from build123d import *

# Parameters (mm, degrees)
SKETCH_1_R      = 1.3
SKETCH_1_R_2    = 4
SKETCH_1_R_3    = 1.925
SKETCH_1_R_4    = 3.85
EXTRUDE_1_DEPTH = 1.5


with BuildPart() as part:
    # 草圖1 → 填料-伸長1 (new body)
    with BuildSketch(Plane(origin=(0, 0, 0), x_dir=(0, 0, -1), z_dir=(1, 0, 0))):
        with BuildLine():
            ThreePointArc((111.555989952, -8.572011863), (6.374730125, -10.137132711), (-98.230068302, -21.244930328))
            ThreePointArc((-98.230068302, -21.244930328), (-123.67575498, -2.873316644), (-103.541794939, 21.20204032))
            ThreePointArc((-103.541794939, 21.20204032), (5.082777822, 20.871677912), (113.584507189, 15.696576829))
            ThreePointArc((113.584507189, 15.696576829), (123.827345593, 3.028727453), (112.406990492, -8.588743688))
            ThreePointArc((112.406990492, -8.588743688), (111.981133536, -8.59851924), (111.555989952, -8.572011863))
        make_face()
        with Locations((-102.143981395, 6.633331517)):
            Circle(SKETCH_1_R, mode=Mode.SUBTRACT)
        with Locations((-108.643981395, 0.133331517)):
            Circle(SKETCH_1_R, mode=Mode.SUBTRACT)
        with Locations((-102.143981395, -6.366668483)):
            Circle(SKETCH_1_R, mode=Mode.SUBTRACT)
        with Locations((-95.643981395, 0.133331517)):
            Circle(SKETCH_1_R, mode=Mode.SUBTRACT)
        with Locations((-102.143981395, 0.133331517)):
            Circle(SKETCH_1_R_2, mode=Mode.SUBTRACT)
        with Locations((35.001055541, 5.982881827)):
            Circle(SKETCH_1_R_3, mode=Mode.SUBTRACT)
        with Locations((-44.432813653, 4.686665047)):
            Circle(SKETCH_1_R_3, mode=Mode.SUBTRACT)
        with Locations((111.605339346, 3.621333032)):
            Circle(SKETCH_1_R_4, mode=Mode.SUBTRACT)
    extrude(amount=EXTRUDE_1_DEPTH)


solid = part.part
Geometry check sheet. Reference: the model listing, model coordinates, mm. A direction names the side the tool comes from. Round coordinates to 2 decimals unless told otherwise and drop trailing zeros. Loops run counter-clockwise (first coordinate to the right, second up) from the corner with the lowest first, then second, coordinate; pieces in that order, holes last.
Item 1: Cross-section at C-C on y = -17.5. Record the boundary of the cut face in (x, z).
Item 2: Mould release check, pull along Z, two halves, no side actions. Record for faces 1 (the cylindrical face through (0.74, 0.31, 106.14)), 2 (the flat face through (0, 5, 26)), 3 (the cylindrical face through (0.74, 3.278, -123.837)): pulls with the +Z half, pulls with the -Z half, needs draft (parallel to the pull), parting line crosses it, or undercut.
Item 3: Thickness scan on line 1 (Z direction, x = 0.3, y = -0.5); line 2 (Z direction, x = 1.35, y = -1); line 3 (Z direction, x = 0.2, y = -2). Record the ranges inside material, lowest first.
Item 4: Gauge pin test, flat ends, axial feed: pin 1 (6 mm diameter, centred on y = -1.5, z = -66.5, fed in from -X); pin 2 (2.5 mm diameter, centred on y = 6.63, z = 102.14, fed in from -X). Record the tip position at first contact, or that the pin passes through.
Item 5: Cross-section at B-B on z = -45. Record the boundary of the cut face in (x, y), then the cut area to 3 significant figures.
Item 6: Cross-section at A-A on x = 0.95. Count the separate pieces of the cut face and the enclosed holes in it, then the cut area to 4 significant figures.
Item 7: Access from +Z, -Z, +X, -X, +Y, -Y to the whole of each face (thin tool, end or side, straight path). Record for faces 4 (the cylindrical face through (0.74, 5.265, 42.597)), 5 (the cylindrical face through (0.74, 20.91, -3.56)), 6 (the cylindrical face through (0.74, -10.05, -7.85)).
Answer sheet:
1. outline: (0, 71.58) - (1.5, 71.58) - (1.5, 115.08) - (0, 115.08) - close
2. face 1: undercut
2. face 2: needs draft
2. face 3: pulls with the -Z half
3. line 1: z = -123.13 to 94.51, 96.78 to 98.19, 106.09 to 107.51, 109.78 to 123.84
3. line 2: z = -122.94 to 95.01, 96.28 to 98.31, 105.98 to 108.01, 109.28 to 123.83
3. line 3: z = -122.47 to 98.76, 105.53 to 123.77
4. pin 1: stops at x = 0
4. pin 2: passes through
5. outline: (0, -8.45) - (1.5, -8.45) - (1.5, 19.53) - (0, 19.53) - close
5. area: 42.0 mm2
6. separate pieces: 1
6. enclosed holes: 8
6. area: 7,665 mm2
7. face 4: +X, -X
7. face 5: +X, -X, +Y
7. face 6: +X, -X, -Y
